Study the drawing (mm; zero at the part's minimum x, y, z) and answer. A direction names the side the tool comes from. Coordinates: 2 decimals unless noted, no trailing zeros. Loops run counter-clockwise (first coordinate to the right, second up) from the corner with the lowest first, then second, coordinate; pieces in that order, holes last. Notation, with made-up numbers: (-32, -26) - (-19, -26) arc R4 cw to (-19, -21) - close; hole circle Ø11 at (-24.75, 26.25). An arc over 180 degrees is marked (long way). Write each question's results on one line, items separated by ' | '. Start each with the question number.
(1) For the marked faces 1, 2 and 3, determine the directions among +Z, -Z, +X, -X, +Y, -Y from which every point of the face is accessible in a straight line to the end or side of a thin tool.
(2) Find section B-B on z = 3.4. Determine the outline of the cut face in (x, y).
(3) Find section D-D on x = 4.5. Determine the outline of the cut face in (y, z).
(4) Determine the mould class of the marked faces 4, 5, 6 and 7 for opening direction X: released by +X, released by -X, zero draft, split by the parting line, or undercut.
(5) Find section A-A on y = 8.25. Determine the outline of the cut face in (x, z).
(6) Given pin 1 Ø1.5 at (x, z) = (4, 3) entering from +Y; pin 2 Ø1 at (x, y) = (8, 6) entering from +Z, each flat-ended and moving along its own axis, determine where each tip first touches the part or whether it passes through.
(7) Consider line 1 (X direction, y = 4, z = 0.5); line 2 (Y direction, x = 7, z = 1.7) (1 decimal); line 3 (Y direction, x = 9.75, z = 0.8). Determine where each line is inside the solid, lowest interval first. Write a range as from..to.
(8) Find section C-C on x = 8.5. Determine the outline of the cut face in (y, z) (1 decimal), then the cut area to 3 significant figures.
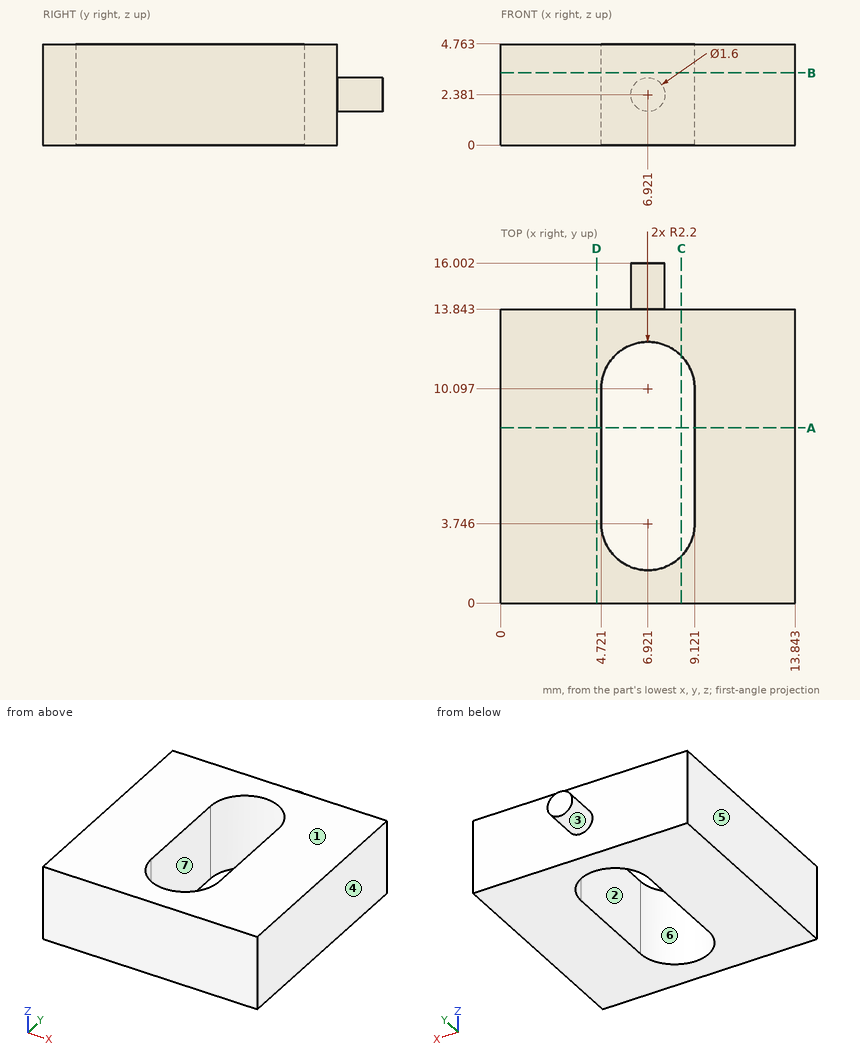
Values:
1) face 1: +Z, +X, -X, +Y, -Y | face 2: +Z, -Z | face 3: +Y
2) outline: (0, 0) - (13.84, 0) - (13.84, 13.84) - (0, 13.84) - close; hole (4.72, 3.75) arc R2.2 ccw to (9.12, 3.75) - (9.12, 10.1) arc R2.2 ccw to (4.72, 10.1) - close
3) outline: (0, 0) - (13.84, 0) - (13.84, 4.76) - (0, 4.76) - close
4) face 4: released by +X | face 5: released by -X | face 6: undercut | face 7: undercut
5) outline: (0, 0) - (4.72, 0) - (4.72, 4.76) - (0, 4.76) - close; (9.12, 0) - (13.84, 0) - (13.84, 4.76) - (9.12, 4.76) - close
6) pin 1: stops at y = 13.84 | pin 2: passes through
7) line 1: x = 0..4.72, 9.12..13.84 | line 2: y = 0..1.5, 12.3..16 | line 3: y = 0..13.84
8) outline: (0, 0) - (2.2, 0) - (2.2, 4.8) - (0, 4.8) - close; (11.6, 0) - (13.8, 0) - (13.8, 4.8) - (11.6, 4.8) - close | area: 21.1 mm²
